from build123d import *

# Parameters (mm, degrees)
SKETCH_1_W      = 114
SKETCH_1_H      = 34
SKETCH_1_R      = 3
SKETCH_1_R_2    = 1.7
EXTRUDE_1_DEPTH = 2


with BuildPart() as part:
    # 草图1 → 凸台-拉伸1 (new, symmetric)
    with BuildSketch(Plane.XY):
        with Locations((40, 0)):
            Rectangle(SKETCH_1_W, SKETCH_1_H)
        Circle(SKETCH_1_R, mode=Mode.SUBTRACT)
        with Locations((80, 0)):
            Circle(SKETCH_1_R_2, mode=Mode.SUBTRACT)
    extrude(amount=EXTRUDE_1_DEPTH, both=True)


solid = part.part
For this review, take the finished solid that the model builds, in its own axes (mm). Give positions to 0.01 mm unless a question says otherwise; leave off trailing zeros. Order: outer loops, then holes, each group sorted by start corner. A loop starts at its lowest first (then second) coordinate and runs counter-clockwise, first axis right, second up. Notation, with made-up numbers: (-12, 26) - (3, 26) arc R17 ccw to (3, 57) - close; hole circle Ø8 at (49.25, 10). An arc over 180 degrees is marked (long way). Answer as a JSON object with one key per item and string values. Group by question number.
Item 1: Clearance check with a flat-ended pin moving along its axis: pin 1 Ø2 at (x, y) = (80, 0) entering from -Z. State where the tip first meets the part, or that it passes through.
Item 2: Take a section at B-B on x = 0. Give the boundary of the cut face in (y, z).
Item 3: Take a section at A-A on y = 0. Give the boundary of the cut face in (x, z).
Item 4: Draft analysis for pull direction Y (two halves, no side actions). For faces 1 (the flat face through (39, 17, 0)), 2 (the cylindrical face through (-3, 0, 0)), 3 (the flat face through (39, 0, -2)), 4 (the cylindrical face through (78.3, 0.07, -0.03)), state which applies: pulls with the +Y half, pulls with the -Y half, needs draft (parallel to the pull), parting line crosses it, or undercut.
Item 5: Wall thickness on line 1 along Y through (x, z) = (80, 1.2); line 2 along Y through (x, z) = (-2, -0.7): over which ranges is each line inside the solid? List them lowest first.
Item 6: Take a section at C-C on x = 80. Give the boundary of the cut face in (y, z), and give its area (3 significant figures).
Reported:
{
 "1": {"pin 1": "through"},
 "2": {"outline": "(-17, -2) - (-3, -2) - (-3, 2) - (-17, 2) - close; (3, -2) - (17, -2) - (17, 2) - (3, 2) - close"},
 "3": {"outline": "(-17, -2) - (-3, -2) - (-3, 2) - (-17, 2) - close; (3, -2) - (78.3, -2) - (78.3, 2) - (3, 2) - close; (81.7, -2) - (97, -2) - (97, 2) - (81.7, 2) - close"},
 "4": {"face 1": "pulls with the +Y half", "face 2": "undercut", "face 3": "needs draft", "face 4": "undercut"},
 "5": {"line 1": "-17 to -1.7, 1.7 to 17", "line 2": "-17 to -2.24, 2.24 to 17"},
 "6": {"outline": "(-17, -2) - (-1.7, -2) - (-1.7, 2) - (-17, 2) - close; (1.7, -2) - (17, -2) - (17, 2) - (1.7, 2) - close", "area": "122 mm^2"}
}
